Geometry check sheet. Reference: drawing and pictorial views, mm from the part's lowest x, y, z. A direction names the side the tool comes from. Give positions to 0.01 mm unless a question says otherwise; leave off trailing zeros. Loops run counter-clockwise (first coordinate to the right, second up) from the corner with the lowest first, then second, coordinate; pieces in that order, holes last. Notation, with made-up numbers: M 10,15.5 L 38,15.5 A19 cw 38,44.5 Z; hole C 86,43.25 d10. An arc over 180 degrees is marked long. Use CSV: the item, a comma, the result in double quotes.
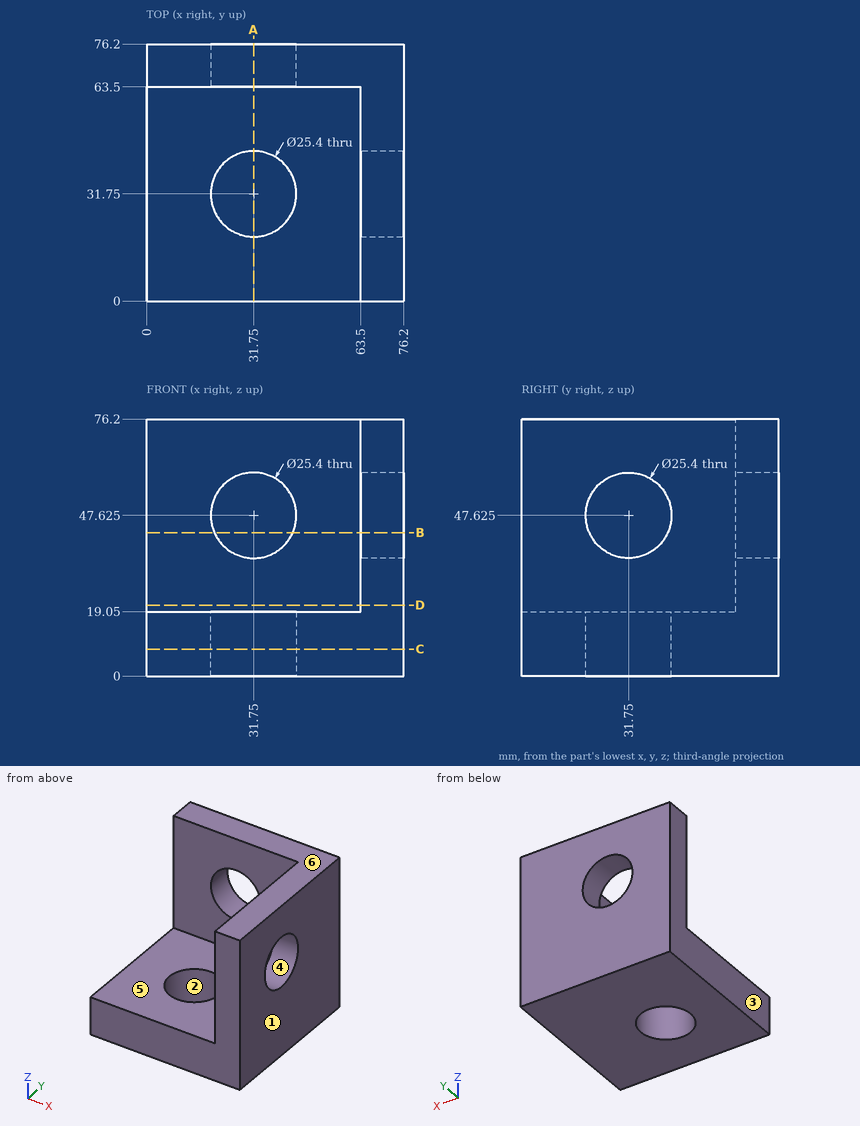
(1) Tool access check on the marked faces 5 and 6. Record the directions out of +Z, -Z, +X, -X, +Y, -Y that give a thin tool (end or side, any length) a straight path to the whole face; none if there is none.
Calculated:
face 5,"+Z, -X, -Y"
face 6,"+Z, +X, -X, +Y, -Y"
(2) Scan lines: L1, parallel to Y at x = 31, z = 14; L2, parallel to Z at x = 31, y = 69; L3, parallel to Z at x = 7.5, y = 13. Record each from-to range of solid material in increasing order. Write a range as from..to.
Calculated:
L1,"y = 0..19.07, 44.43..76.2"
L2,"z = 0..34.95, 60.3..76.2"
L3,"z = 0..19.05"
(3) Section check D-D on z = 21. Record the cut outline in (x, y).
Calculated:
outline,"M 0,63.5 L 63.5,63.5 L 63.5,0 L 76.2,0 L 76.2,76.2 L 0,76.2 Z"
(4) Mould release check, pull along X, two halves, no side actions. Record for the marked faces 1, 2, 3 and 4: released by +X, released by -X, zero draft, split by the parting line, or undercut.
Calculated:
face 1,"released by +X"
face 2,"undercut"
face 3,"released by -X"
face 4,"zero draft"
(5) Section check A-A on x = 31.75. Record the cut outline in (y, z) (3 decimals), plus the area to 3 significant figures.
Calculated:
outline,"M 0,0 L 19.05,0 L 19.05,19.05 L 0,19.05 Z; M 44.45,0 L 76.2,0 L 76.2,34.925 L 63.5,34.925 L 63.5,19.05 L 44.45,19.05 Z; M 63.5,60.325 L 76.2,60.325 L 76.2,76.2 L 63.5,76.2 Z"
area,"1,370 mm²"
(6) Section check C-C on z = 8. Record the cut outline in (x, y).
Calculated:
outline,"M 0,0 L 76.2,0 L 76.2,76.2 L 0,76.2 Z; hole C 31.75,31.75 d25.4"
(7) Section check B-B on z = 42.5. Record the cut outline in (x, y), plus the area to 3 significant figures.
Calculated:
outline,"M 0,63.5 L 20.13,63.5 L 20.13,76.2 L 0,76.2 Z; M 43.37,63.5 L 63.5,63.5 L 63.5,43.37 L 76.2,43.37 L 76.2,76.2 L 43.37,76.2 Z; M 63.5,0 L 76.2,0 L 76.2,20.13 L 63.5,20.13 Z"
area,"1,180 mm²"
(8) Depth check by flat-ended pin: pin 1 Ø19 at (x, y) = (43, 34) entering from +Z; pin 2 Ø23 at (x, z) = (31.75, 47.625) entering from -Y; pin 3 Ø8 at (y, z) = (43, 64) entering from -X; pin 4 Ø6 at (x, z) = (57, 27.5) entering from -Y. Enter the tip coordinate at first touch or a pass-through.
Calculated:
pin 1,"stops at z = 19.05"
pin 2,"passes through"
pin 3,"stops at x = 63.5"
pin 4,"stops at y = 63.5"
